```python
from build123d import *

# Parameters (mm, degrees)
F0_W      = 115
F0_H      = 75
F1_DEPTH  = 2.5
F2_W      = 115
F2_H      = 23.5
F3_DEPTH  = 3
F4_W      = 40
F4_H      = 10
F5_DEPTH  = 2.5
F6_W      = 23.5
F6_H      = 20
F7_DEPTH  = 2.5
F8_W      = 23.5
F8_H      = 20
F9_DEPTH  = 2.5
F10_W     = 2.5
F10_H     = 15
F10_H_2   = 58
F11_DEPTH = 2.5
F12_W     = 2.5
F12_H     = 15
F12_H_2   = 58
F13_DEPTH = 2.5
F14_W     = 57.15
F14_H     = 78
F15_DEPTH = 25.4
F16_R     = 25.4
F17_DEPTH = 78
F19_DEPTH = 1
F20_DEPTH = 1
F18_W     = 2
F18_H     = 70
F21_DEPTH = 57.15


with BuildPart() as f1:
    # F0 (on Front) → F1 (new body)
    with BuildSketch(Plane.XZ):
        Rectangle(F0_W, F0_H)
    extrude(amount=-F1_DEPTH)

    # F2 (on face) → F3 (join)
    with BuildSketch(Plane(origin=(0, 0, -37.5), x_dir=(1, 0, 0), z_dir=(0, 0, -1))):
        with Locations((0, 9.25)):
            Rectangle(F2_W, F2_H)
    extrude(amount=F3_DEPTH)

    # F4 (on face) → F5 (join)
    with BuildSketch(Plane.XZ.offset(21)):
        Polygon((-57.5, -5.5), (-57.5, -40.5), (-47.5, -40.5), (-47.5, -30.5), (-47.5, -5.5), align=None)
        with Locations((-27.5, -35.5)):
            Rectangle(F4_W, F4_H)
        Polygon((-7.5, -30.5), (-7.5, -40.5), (0, -40.5), (0, -5.5), (-7.5, -5.5), align=None)
        Polygon((0, -5.5), (0, -40.5), (7.5, -40.5), (7.5, -30.5), (7.5, -5.5), align=None)
        with Locations((27.5, -35.5)):
            Rectangle(F4_W, F4_H)
        Polygon((47.5, -30.5), (47.5, -40.5), (57.5, -40.5), (57.5, -5.5), (47.5, -5.5), align=None)
    extrude(amount=-F5_DEPTH)

    # F6 (on face) → F7 (join)
    with BuildSketch(Plane(origin=(-57.5, 0, 0), x_dir=(0, -1, 0), z_dir=(-1, 0, 0))):
        with Locations((9.25, -30.5)):
            Rectangle(F6_W, F6_H)
    extrude(amount=F7_DEPTH)

    # F8 (on face) → F9 (join)
    with BuildSketch(Plane.YZ.offset(57.5)):
        with Locations((-9.25, -30.5)):
            Rectangle(F8_W, F8_H)
    extrude(amount=F9_DEPTH)

    # F10 (on face) → F11 (join)
    with BuildSketch(Plane.YZ.offset(57.5)):
        with Locations((-19.75, -13)):
            Rectangle(F10_W, F10_H)
        with Locations((1.25, 8.5)):
            Rectangle(F10_W, F10_H_2)
    extrude(amount=F11_DEPTH)

    # F12 (on face) → F13 (join)
    with BuildSketch(Plane(origin=(-57.5, 0, 0), x_dir=(0, -1, 0), z_dir=(-1, 0, 0))):
        with Locations((19.75, -13)):
            Rectangle(F12_W, F12_H)
        with Locations((-1.25, 8.5)):
            Rectangle(F12_W, F12_H_2)
    extrude(amount=F13_DEPTH)

    # F14 (on face) → F15 (join)
    with BuildSketch(Plane(origin=(0, 2.5, 0), x_dir=(-1, 0, 0), z_dir=(0, 1, 0))):
        with Locations((0, -1.5)):
            Rectangle(F14_W, F14_H)
    extrude(amount=F15_DEPTH)

    # F16 (on face) → F17 (cut)
    with BuildSketch(Plane.XY.offset(37.5)):
        with Locations((0, 27.9)):
            Circle(F16_R)
    extrude(amount=-F17_DEPTH, mode=Mode.SUBTRACT)

    # F6 (on face) → F19 (join)
    with BuildSketch(Plane(origin=(-57.5, 0, 0), x_dir=(0, -1, 0), z_dir=(-1, 0, 0))):
        with Locations((9.25, -30.5)):
            Rectangle(F6_W, F6_H)
    extrude(amount=-F19_DEPTH)

    # F8 (on face) → F20 (join)
    with BuildSketch(Plane.YZ.offset(57.5)):
        with Locations((-9.25, -30.5)):
            Rectangle(F8_W, F8_H)
    extrude(amount=-F20_DEPTH)

    # F18 (on face) → F21 (cut)
    with BuildSketch(Plane.YZ.offset(28.575)):
        with Locations((23.9, -1.5)):
            Rectangle(F18_W, F18_H)
    extrude(amount=-F21_DEPTH, mode=Mode.SUBTRACT)


solid = f1.part
```
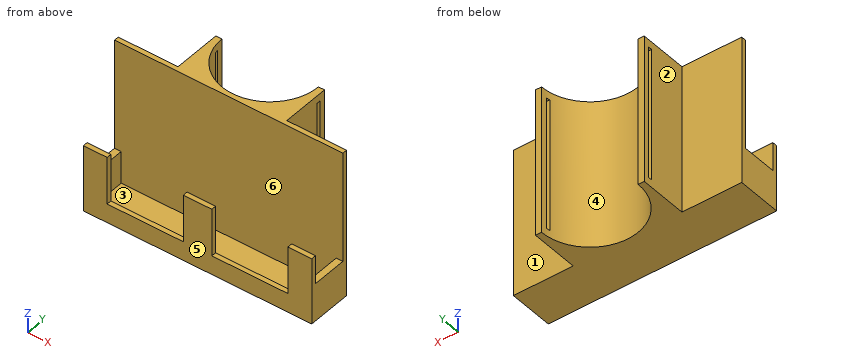
Part model, mm, in its own coordinate system. Face numbers are marked on the shaded views. A direction names the side the tool comes from. Coordinates: 2 decimals unless noted, no trailing zeros. Write each loop counter-clockwise with the first axis right and the second up, starting at its lowest first coordinate (ties: lowest second). Pieces come first, ordered by that corner, then holes.
Item 1: Which spindle directions (+Z, -Z, +X, -X, +Y, -Y) get a long thin tool onto all of the face, cutting with end or side? Do the marked faces 1, 2 and 3. Say none if no direction does.
Item 2: Slice it at C-C (x = 0). Write the cut outline in (y, z).
Item 3: Pin check, flat tips, straight feed: pin 1 (2 mm diameter, centred on x = -51, y = -19.5, fed in from +Z); pin 2 (1 mm diameter, centred on x = -15, z = -10, fed in from -Y); pin 3 (6 mm diameter, centred on x = -44, z = -31, fed in from +Y). Stop position of each tip, or through.
Item 4: Slice it at B-B (z = -24). Count the separate pieces of the cut face and the enclosed holes in it, and give its area (3 significant figures).
Item 5: Mould opens along Y. For the marked faces 4, 5 and 6 say: released by +Y, released by -Y, zero draft, split by the parting line, or undercut.
Item 6: Slice it at D-D (y = -4). Write the cut outline in (x, z).
Item 7: Probe line 1 (X direction, y = -5.5, z = -25.5); line 2 (Z direction, x = 46.5, y = -14); line 3 (Y direction, x = -51, z = -13.5). List the from-to ranges inside material, lowest first.
Item 8: Slice it at A-A (z = 27). Write the cut outline in (x, y) (3 decimals).
Results found:
1. face 1: +Z, -Z, +X, +Y
1. face 2: +Z, -Z, -X, +Y
1. face 3: +Z
2. outline: (-21, -40.5) - (2.5, -40.5) - (2.5, 37.5) - (0, 37.5) - (0, -37.5) - (-18.5, -37.5) - (-18.5, -5.5) - (-21, -5.5) - close
3. pin 1: stops at z = -5.5
3. pin 2: stops at y = 0
3. pin 3: stops at y = 2.5
4. separate pieces: 4
4. enclosed holes: 0
4. area: 954 mm2
5. face 4: released by +Y
5. face 5: released by -Y
5. face 6: undercut
6. outline: (-60, -40.5) - (60, -40.5) - (60, -20.5) - (56.5, -20.5) - (56.5, -37.5) - (-56.5, -37.5) - (-56.5, -20.5) - (-60, -20.5) - close
7. line 1: x = -60 to -56.5, 56.5 to 60
7. line 2: z = -40.5 to -37.5
7. line 3: y = -21 to -18.5, 0 to 2.5
8. outline: (-60, 0) - (60, 0) - (60, 2.5) - (28.575, 2.5) - (28.575, 22.9) - (24.903, 22.9) arc R25.4 cw to (-24.903, 22.9) - (-28.575, 22.9) - (-28.575, 2.5) - (-60, 2.5) - close; (-28.575, 24.9) - (-25.222, 24.9) arc R25.4 cw to (-25.4, 27.9) - (-28.575, 27.9) - close; (25.222, 24.9) - (28.575, 24.9) - (28.575, 27.9) - (25.4, 27.9) arc R25.4 cw to start
